from build123d import *

# Parameters (mm, degrees)
SKETCH1_W                    = 609.6
SKETCH1_H                    = 609.6
SKETCH1_R                    = 76.2
BOSS_EXTRUDE1_DEPTH          = 6.35
SKETCH3_R                    = 3.175
CUT_EXTRUDE1_DEPTH           = 6.35
LPATTERN1_COUNT              = 5
LPATTERN1_PITCH              = 25.4
CIRPATTERN1_COUNT            = 4
CIRPATTERN1_COPY_1_SKETCH_R  = 3.175
CIRPATTERN1_COPY_1_DEPTH     = 6.35
CIRPATTERN1_COPY_2_SKETCH_R  = 3.175
CIRPATTERN1_COPY_2_DEPTH     = 6.35
CIRPATTERN1_COPY_3_SKETCH_R  = 3.175
CIRPATTERN1_COPY_3_DEPTH     = 6.35
CIRPATTERN1_COPY_4_SKETCH_R  = 3.175
CIRPATTERN1_COPY_4_DEPTH     = 6.35
CIRPATTERN1_COPY_5_SKETCH_R  = 3.175
CIRPATTERN1_COPY_5_DEPTH     = 6.35
CIRPATTERN1_COPY_6_SKETCH_R  = 3.175
CIRPATTERN1_COPY_6_DEPTH     = 6.35
CIRPATTERN1_COPY_7_SKETCH_R  = 3.175
CIRPATTERN1_COPY_7_DEPTH     = 6.35
CIRPATTERN1_COPY_8_SKETCH_R  = 3.175
CIRPATTERN1_COPY_8_DEPTH     = 6.35
CIRPATTERN1_COPY_9_SKETCH_R  = 3.175
CIRPATTERN1_COPY_9_DEPTH     = 6.35
CIRPATTERN1_COPY_10_SKETCH_R = 3.175
CIRPATTERN1_COPY_10_DEPTH    = 6.35
CIRPATTERN1_COPY_11_SKETCH_R = 3.175
CIRPATTERN1_COPY_11_DEPTH    = 6.35
CIRPATTERN1_COPY_12_SKETCH_R = 3.175
CIRPATTERN1_COPY_12_DEPTH    = 6.35


with BuildPart() as part:
    # Sketch1 → Boss-Extrude1 (new body)
    with BuildSketch(Plane.XY):
        Rectangle(SKETCH1_W, SKETCH1_H)
        Circle(SKETCH1_R, mode=Mode.SUBTRACT)
    extrude(amount=-BOSS_EXTRUDE1_DEPTH)

    # Sketch3 → Cut-Extrude1 (cut)
    with BuildSketch(Plane.XY):
        with Locations((-127, 0)):
            Circle(SKETCH3_R)
        with Locations((-127, 25.4)):
            Circle(SKETCH3_R)
        with Locations((-127, -25.4)):
            Circle(SKETCH3_R)
    cut_extrude1 = extrude(amount=-CUT_EXTRUDE1_DEPTH, mode=Mode.SUBTRACT)

    # LPattern1: Cut-Extrude1 ×5
    with Locations(*[(-i * LPATTERN1_PITCH, 0, 0) for i in range(1, LPATTERN1_COUNT)]):
        add(cut_extrude1, mode=Mode.SUBTRACT)

    # CirPattern1: Cut-Extrude1 ×4 about axis
    cirpattern1_axis = Axis((0, 0, 0), (0, 0, 1))
    for i in range(1, CIRPATTERN1_COUNT):
        add(cut_extrude1.rotate(cirpattern1_axis, i * 360 / CIRPATTERN1_COUNT), mode=Mode.SUBTRACT)

    # CirPattern1 copy 1 sketch → CirPattern1 copy 1 (cut)
    with BuildSketch(Plane(origin=(0, -25.4, 0), x_dir=(0, 1, 0), z_dir=(0, 0, 1))):
        with Locations((-127, 0)):
            Circle(CIRPATTERN1_COPY_1_SKETCH_R)
        with Locations((-127, 25.4)):
            Circle(CIRPATTERN1_COPY_1_SKETCH_R)
        with Locations((-127, -25.4)):
            Circle(CIRPATTERN1_COPY_1_SKETCH_R)
    extrude(amount=-CIRPATTERN1_COPY_1_DEPTH, mode=Mode.SUBTRACT)

    # CirPattern1 copy 2 sketch → CirPattern1 copy 2 (cut)
    with BuildSketch(Plane(origin=(25.4, 0, 0), x_dir=(-1, 0, 0), z_dir=(0, 0, 1))):
        with Locations((-127, 0)):
            Circle(CIRPATTERN1_COPY_2_SKETCH_R)
        with Locations((-127, 25.4)):
            Circle(CIRPATTERN1_COPY_2_SKETCH_R)
        with Locations((-127, -25.4)):
            Circle(CIRPATTERN1_COPY_2_SKETCH_R)
    extrude(amount=-CIRPATTERN1_COPY_2_DEPTH, mode=Mode.SUBTRACT)

    # CirPattern1 copy 3 sketch → CirPattern1 copy 3 (cut)
    with BuildSketch(Plane(origin=(0, 25.4, 0), x_dir=(0, -1, 0), z_dir=(0, 0, 1))):
        with Locations((-127, 0)):
            Circle(CIRPATTERN1_COPY_3_SKETCH_R)
        with Locations((-127, 25.4)):
            Circle(CIRPATTERN1_COPY_3_SKETCH_R)
        with Locations((-127, -25.4)):
            Circle(CIRPATTERN1_COPY_3_SKETCH_R)
    extrude(amount=-CIRPATTERN1_COPY_3_DEPTH, mode=Mode.SUBTRACT)

    # CirPattern1 copy 4 sketch → CirPattern1 copy 4 (cut)
    with BuildSketch(Plane(origin=(0, -50.8, 0), x_dir=(0, 1, 0), z_dir=(0, 0, 1))):
        with Locations((-127, 0)):
            Circle(CIRPATTERN1_COPY_4_SKETCH_R)
        with Locations((-127, 25.4)):
            Circle(CIRPATTERN1_COPY_4_SKETCH_R)
        with Locations((-127, -25.4)):
            Circle(CIRPATTERN1_COPY_4_SKETCH_R)
    extrude(amount=-CIRPATTERN1_COPY_4_DEPTH, mode=Mode.SUBTRACT)

    # CirPattern1 copy 5 sketch → CirPattern1 copy 5 (cut)
    with BuildSketch(Plane(origin=(50.8, 0, 0), x_dir=(-1, 0, 0), z_dir=(0, 0, 1))):
        with Locations((-127, 0)):
            Circle(CIRPATTERN1_COPY_5_SKETCH_R)
        with Locations((-127, 25.4)):
            Circle(CIRPATTERN1_COPY_5_SKETCH_R)
        with Locations((-127, -25.4)):
            Circle(CIRPATTERN1_COPY_5_SKETCH_R)
    extrude(amount=-CIRPATTERN1_COPY_5_DEPTH, mode=Mode.SUBTRACT)

    # CirPattern1 copy 6 sketch → CirPattern1 copy 6 (cut)
    with BuildSketch(Plane(origin=(0, 50.8, 0), x_dir=(0, -1, 0), z_dir=(0, 0, 1))):
        with Locations((-127, 0)):
            Circle(CIRPATTERN1_COPY_6_SKETCH_R)
        with Locations((-127, 25.4)):
            Circle(CIRPATTERN1_COPY_6_SKETCH_R)
        with Locations((-127, -25.4)):
            Circle(CIRPATTERN1_COPY_6_SKETCH_R)
    extrude(amount=-CIRPATTERN1_COPY_6_DEPTH, mode=Mode.SUBTRACT)

    # CirPattern1 copy 7 sketch → CirPattern1 copy 7 (cut)
    with BuildSketch(Plane(origin=(0, -76.2, 0), x_dir=(0, 1, 0), z_dir=(0, 0, 1))):
        with Locations((-127, 0)):
            Circle(CIRPATTERN1_COPY_7_SKETCH_R)
        with Locations((-127, 25.4)):
            Circle(CIRPATTERN1_COPY_7_SKETCH_R)
        with Locations((-127, -25.4)):
            Circle(CIRPATTERN1_COPY_7_SKETCH_R)
    extrude(amount=-CIRPATTERN1_COPY_7_DEPTH, mode=Mode.SUBTRACT)

    # CirPattern1 copy 8 sketch → CirPattern1 copy 8 (cut)
    with BuildSketch(Plane(origin=(76.2, 0, 0), x_dir=(-1, 0, 0), z_dir=(0, 0, 1))):
        with Locations((-127, 0)):
            Circle(CIRPATTERN1_COPY_8_SKETCH_R)
        with Locations((-127, 25.4)):
            Circle(CIRPATTERN1_COPY_8_SKETCH_R)
        with Locations((-127, -25.4)):
            Circle(CIRPATTERN1_COPY_8_SKETCH_R)
    extrude(amount=-CIRPATTERN1_COPY_8_DEPTH, mode=Mode.SUBTRACT)

    # CirPattern1 copy 9 sketch → CirPattern1 copy 9 (cut)
    with BuildSketch(Plane(origin=(0, 76.2, 0), x_dir=(0, -1, 0), z_dir=(0, 0, 1))):
        with Locations((-127, 0)):
            Circle(CIRPATTERN1_COPY_9_SKETCH_R)
        with Locations((-127, 25.4)):
            Circle(CIRPATTERN1_COPY_9_SKETCH_R)
        with Locations((-127, -25.4)):
            Circle(CIRPATTERN1_COPY_9_SKETCH_R)
    extrude(amount=-CIRPATTERN1_COPY_9_DEPTH, mode=Mode.SUBTRACT)

    # CirPattern1 copy 10 sketch → CirPattern1 copy 10 (cut)
    with BuildSketch(Plane(origin=(0, -101.6, 0), x_dir=(0, 1, 0), z_dir=(0, 0, 1))):
        with Locations((-127, 0)):
            Circle(CIRPATTERN1_COPY_10_SKETCH_R)
        with Locations((-127, 25.4)):
            Circle(CIRPATTERN1_COPY_10_SKETCH_R)
        with Locations((-127, -25.4)):
            Circle(CIRPATTERN1_COPY_10_SKETCH_R)
    extrude(amount=-CIRPATTERN1_COPY_10_DEPTH, mode=Mode.SUBTRACT)

    # CirPattern1 copy 11 sketch → CirPattern1 copy 11 (cut)
    with BuildSketch(Plane(origin=(101.6, 0, 0), x_dir=(-1, 0, 0), z_dir=(0, 0, 1))):
        with Locations((-127, 0)):
            Circle(CIRPATTERN1_COPY_11_SKETCH_R)
        with Locations((-127, 25.4)):
            Circle(CIRPATTERN1_COPY_11_SKETCH_R)
        with Locations((-127, -25.4)):
            Circle(CIRPATTERN1_COPY_11_SKETCH_R)
    extrude(amount=-CIRPATTERN1_COPY_11_DEPTH, mode=Mode.SUBTRACT)

    # CirPattern1 copy 12 sketch → CirPattern1 copy 12 (cut)
    with BuildSketch(Plane(origin=(0, 101.6, 0), x_dir=(0, -1, 0), z_dir=(0, 0, 1))):
        with Locations((-127, 0)):
            Circle(CIRPATTERN1_COPY_12_SKETCH_R)
        with Locations((-127, 25.4)):
            Circle(CIRPATTERN1_COPY_12_SKETCH_R)
        with Locations((-127, -25.4)):
            Circle(CIRPATTERN1_COPY_12_SKETCH_R)
    extrude(amount=-CIRPATTERN1_COPY_12_DEPTH, mode=Mode.SUBTRACT)


solid = part.part
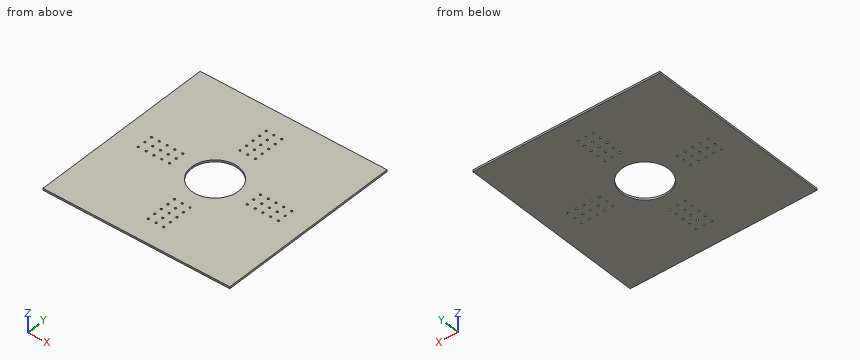
Could you check a few things on this model? Use its own coordinates, in mm. Give positions to 0.01 mm unless a question says otherwise; leave off trailing zeros. Order: outer loops, then holes, each group sorted by start corner. A loop starts at its lowest first (then second) coordinate and runs counter-clockwise, first axis right, second up.
1. I need wall thicknesses on L1, parallel to Y at x = 177.8, z = -1.75 (3 decimals); L2, parallel to X at y = 129.5, z = -3.5. Which ranges of each line are inside material? Lowest first, please.
2. Suppose I cut it at B-B (z = -4.25). Give the number of separate pieces and of enclosed holes in the cut face, plus the area to 3 significant figures.
3. Suppose I cut it at A-A (x = -38). List the corners of the cut face in (y, z) for me.
Solved:
1. L1: y = -304.8 to -28.575, -22.225 to -3.175, 3.175 to 22.225, 28.575 to 304.8
1. L2: x = -304.8 to -27.36, -23.44 to -1.96, 1.96 to 23.44, 27.36 to 304.8
2. separate pieces: 1
2. enclosed holes: 61
2. area: 351,000 mm2
3. outline: (-304.8, -6.35) - (-66.05, -6.35) - (-66.05, 0) - (-304.8, 0) - close; (66.05, -6.35) - (304.8, -6.35) - (304.8, 0) - (66.05, 0) - close
